Check sheet for the drawn part. Datum: minimum x, y, z corner. Units: mm. A direction names the side the tool comes from. Coordinates: 2 decimals unless noted, no trailing zeros. Loops run counter-clockwise (first coordinate to the right, second up) from the corner with the lowest first, then second, coordinate; pieces in that order, holes last. Notation, with made-up numbers: M 16.5,65 L 65.5,65 A21 ccw 65.5,97 Z; hole C 43.25,-35.75 d2. An arc over 180 degrees is marked long. Use CSV: the item, a comma, the result in double quotes. Start each with the question number.
(1) Set-up check for the marked faces 1, 2, 3 and 4: record each of +Z, -Z, +X, -X, +Y, -Y from which the full face is reachable in a straight line by a thin tool's end or side.
(2) Go/stop test with flat-tipped pins: pin 1 Ø14.5 at (x, y) = (23, 22.5) entering from -Z; pin 2 Ø11 at (x, y) = (53.5, 19.5) entering from +Z; pin 3 Ø22.5 at (y, z) = (26, 33) entering from -X; pin 4 Ø1 at (x, z) = (45, 17) entering from -Y. Record where each tip stops, or that it passes through.
(3) Draft check along X on the marked faces 5, 6, 7 and 8. Enter one of: pulls with the +X half, pulls with the -X half, needs draft (parallel to the pull), parting line crosses it, or undercut.
(4) Section check D-D on x = 48. Record the cut outline in (y, z), and give its area (3 significant figures).
(5) Scan lines: line 1 (Z direction, x = 48.5, y = 26); line 2 (X direction, y = 45, z = 41.5); line 3 (Y direction, x = 38, z = 33). Record each from-to range of solid material in increasing order.
(6) Section check A-A on z = 33. Record the cut outline in (x, y).
(7) Section check B-B on y = 26. Record the cut outline in (x, z).
(8) Section check C-C on z = 17. Record the cut outline in (x, y).
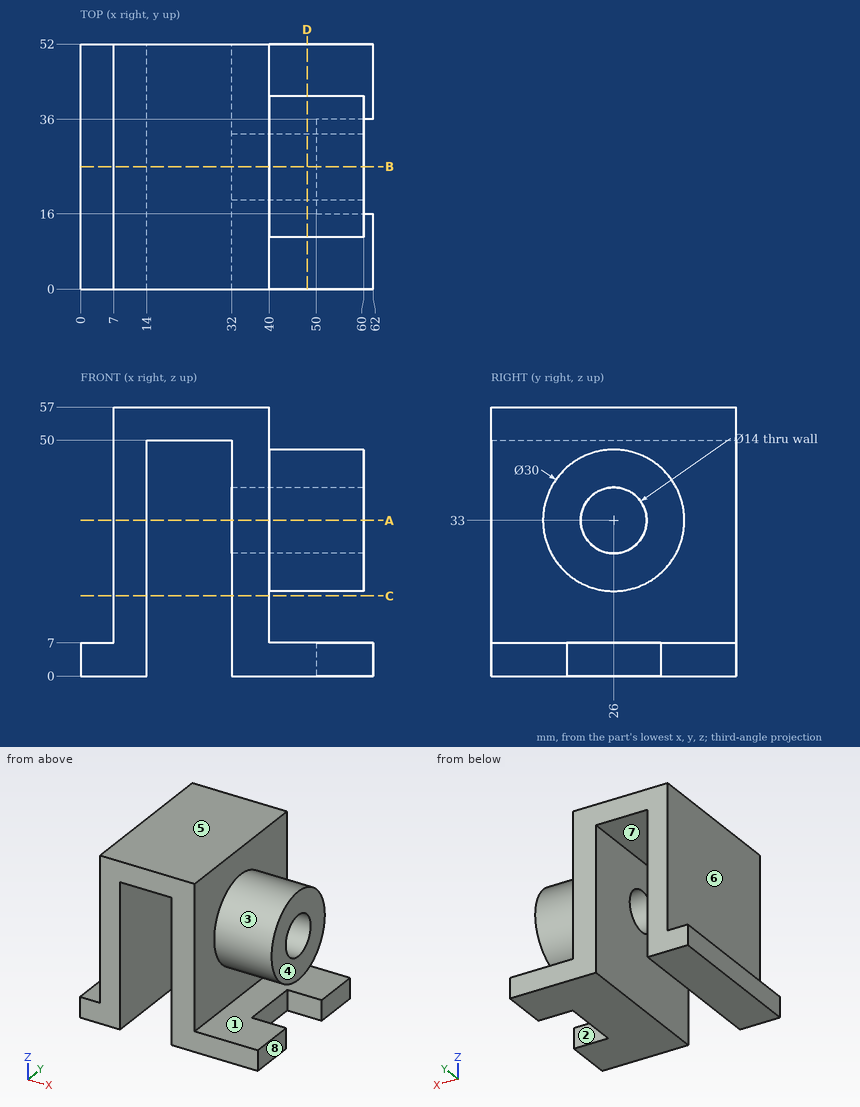
Outcome:
1,face 1,"+X, +Y, -Y"
1,face 2,"-Z, +X"
1,face 3,"+X"
1,face 4,"+Z, +X, +Y, -Y"
2,pin 1,"stops at z = 50"
2,pin 2,"stops at z = 47.97"
2,pin 3,"stops at x = 7"
2,pin 4,"passes through"
3,face 5,"needs draft"
3,face 6,"pulls with the -X half"
3,face 7,"undercut"
3,face 8,"pulls with the +X half"
4,outline,"M 0,0 L 52,0 L 52,7 L 0,7 Z; C 26,33 d30; hole C 26,33 d14"
4,area,"917 mm²"
5,line 1,"z = 0 to 7, 18 to 26, 40 to 48"
5,line 2,"x = 7 to 14, 32 to 40"
5,line 3,"y = 0 to 19, 33 to 52"
6,outline,"M 7,0 L 14,0 L 14,52 L 7,52 Z; M 32,0 L 40,0 L 40,11 L 60,11 L 60,19 L 32,19 Z; M 32,33 L 60,33 L 60,41 L 40,41 L 40,52 L 32,52 Z"
7,outline,"M 0,0 L 14,0 L 14,50 L 32,50 L 32,40 L 60,40 L 60,48 L 40,48 L 40,57 L 7,57 L 7,7 L 0,7 Z; M 32,0 L 50,0 L 50,7 L 40,7 L 40,18 L 60,18 L 60,26 L 32,26 Z"
8,outline,"M 7,0 L 14,0 L 14,52 L 7,52 Z; M 32,0 L 40,0 L 40,52 L 32,52 Z"
